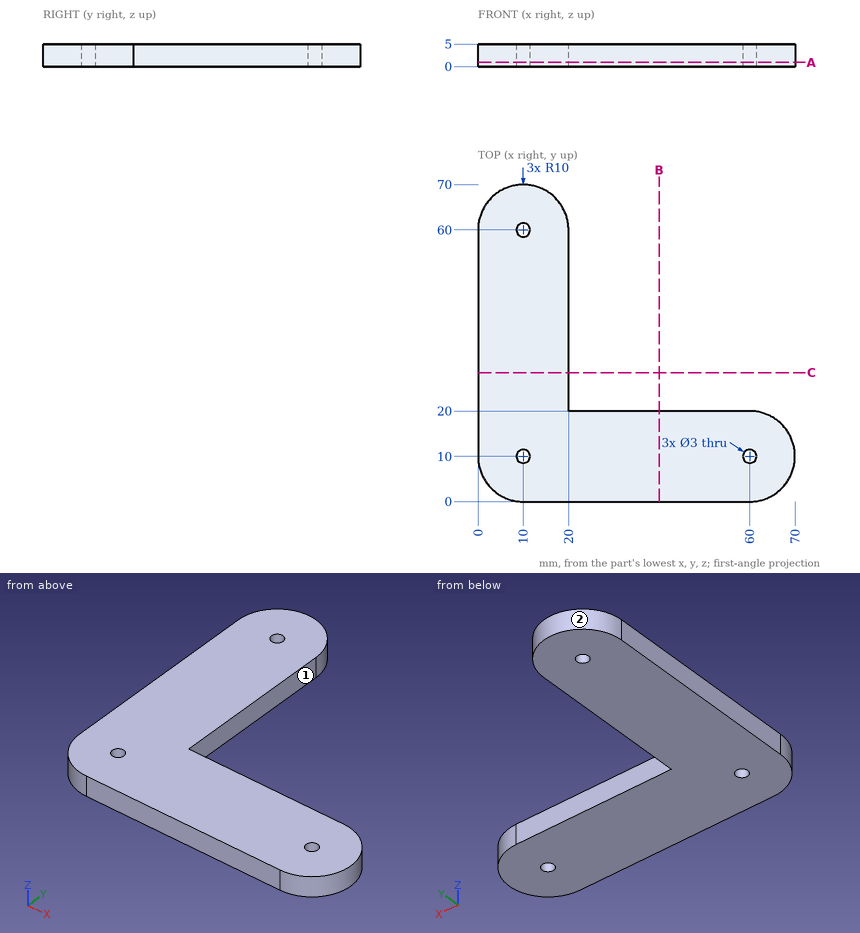
Answer from the drawing. Dimensions are ordinates in mm from the lowest x, y and z of the part. A direction names the side the tool comes from. Round coordinates to 2 decimals unless told otherwise and drop trailing zeros. Loops run counter-clockwise (first coordinate to the right, second up) from the corner with the lowest first, then second, coordinate; pieces in that order, holes last.
Q1. Consider probe 1 along Y at (x, z) = (10, 1.3); probe 2 along X at (y, z) = (35.5, 4.65); probe 3 along Y at (x, z) = (60, 3.3). Determine where each line is inside the solid, lowest interval first.
Q2. Each of these flat-tipped pins is pushed along its axis until it touches: pin 1 (1.5 mm diameter, centred on y = 62, z = 2, fed in from +X); pin 2 (2 mm diameter, centred on y = 7.5, z = 2.5, fed in from +X); pin 3 (2.5 mm diameter, centred on x = 10, y = 10, fed in from +Z); pin 4 (1.5 mm diameter, centred on y = 42.5, z = 2.5, fed in from +X). Where does it stop, or does it pass through?
Q3. Section A-A on z = 0.95 is taken. Write down the section's boundary in (x, y).
Q4. Section B-B on x = 40 is taken. Write down the section's boundary in (y, z).
Q5. Which of the six approach directions +Z, -Z, +X, -X, +Y, -Y give full straight-line access (tool end or side, diameter ignored) to the marked faces 1 and 2?
Output:
1. probe 1: y = 0 to 8.5, 11.5 to 58.5, 61.5 to 70
1. probe 2: x = 0 to 20
1. probe 3: y = 0 to 8.5, 11.5 to 20
2. pin 1: stops at x = 19.92
2. pin 2: stops at x = 69.89
2. pin 3: passes through
2. pin 4: stops at x = 20
3. outline: (0, 10) arc R10 ccw to (10, 0) - (60, 0) arc R10 ccw to (60, 20) - (20, 20) - (20, 60) arc R10 ccw to (0, 60) - close; hole circle Ø3 at (10, 10); hole circle Ø3 at (10, 60); hole circle Ø3 at (60, 10)
4. outline: (0, 0) - (20, 0) - (20, 5) - (0, 5) - close
5. face 1: +Z, -Z, +X, +Y
5. face 2: +Z, -Z, +Y
